For this review, take the finished solid that the model builds, in its own axes (mm). Face numbers are marked on the shaded views. A direction names the side the tool comes from. Round coordinates to 2 decimals unless told otherwise and drop trailing zeros. Write each loop counter-clockwise with the first axis right and the second up, starting at its lowest first coordinate (ties: lowest second). Pieces come first, ordered by that corner, then holes. Notation, with made-up numbers: M 33.5,23 L 39.5,23 A27 ccw 39.5,44 Z; hole C 6.5,59.5 d3. An arc over 180 degrees is marked long. Write each question's results on one line, items separated by ' | '. Start each with the question number.
```python
from build123d import *

# Parameters (mm, degrees)
EXTRUDE1_DEPTH = 7
SHELL1_T       = -1.25
SKETCH2_R      = 2.45
EXTRUDE2_DEPTH = 5.5
EXTRUDE3_REACH = 17.167
SKETCH3_R      = 1.91
EXTRUDE4_REACH = 17.167
SKETCH4_R      = 1.91


with BuildPart() as part:
    # Sketch1 → Extrude1 (new body)
    with BuildSketch(Plane.XY):
        Polygon((-5.45, 6.4), (-7.7, -6.4), (7.7, -6.4), (5.45, 6.4), align=None)
    extrude(amount=EXTRUDE1_DEPTH)

    # Shell1
    shell1_openings = [part.faces().sort_by_distance(p)[0] for p in [
        (0, -6.4, 3.5),
    ]]
    offset(amount=SHELL1_T, openings=shell1_openings, kind=Kind.INTERSECTION)

    # Sketch2 → Extrude2 (add)
    with BuildSketch(Plane(origin=(0, 6.4, 0), x_dir=(1, 0, 0), z_dir=(0, 1, 0))):
        with Locations((0, -3.5)):
            Circle(SKETCH2_R)
    extrude(amount=EXTRUDE2_DEPTH)

    # Sketch3 → Extrude3 (cut, up to next)
    with BuildSketch(Plane(origin=(-6.377928095, 1.121120173, 0), x_dir=(0, 0, 1), z_dir=(-0.984899531, 0.173126871, 0)), mode=Mode.PRIVATE) as extrude3_sk1:
        with Locations((3.5, 1.819815554)):
            Circle(SKETCH3_R)
    extrude3_tool1 = extrude(extrude3_sk1.sketch, amount=-EXTRUDE3_REACH, mode=Mode.PRIVATE) & part.part
    add(extrude3_tool1.solids().sort_by_distance((-6.062869, 2.913456, 3.5))[0], mode=Mode.SUBTRACT)

    # Sketch4 → Extrude4 (cut, up to next)
    with BuildSketch(Plane(origin=(6.377928095, 1.121120173, 0), x_dir=(0, 0, -1), z_dir=(0.984899531, 0.173126871, 0)), mode=Mode.PRIVATE) as extrude4_sk1:
        with Locations((-3.5, 1.819815554)):
            Circle(SKETCH4_R)
    extrude4_tool1 = extrude(extrude4_sk1.sketch, amount=-EXTRUDE4_REACH, mode=Mode.PRIVATE) & part.part
    add(extrude4_tool1.solids().sort_by_distance((6.062869, 2.913456, 3.5))[0], mode=Mode.SUBTRACT)


solid = part.part
```
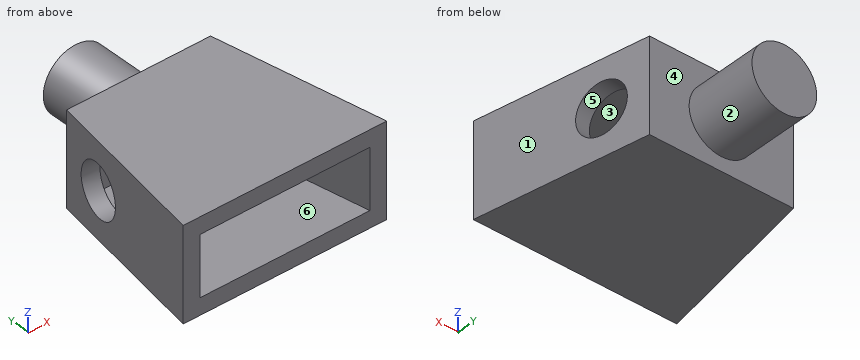
Item 1: Insertion check: P1, Ø4, axis at x = -3, y = 9.5, coming from the -Z side; P2, Ø4, axis at y = 8.5, z = 2, coming from the +X side; P3, Ø2, axis at x = 0, z = 2.5, coming from the -Y side; P4, Ø1, axis at x = 3, y = 8.5, coming from the -Z side. Each pin has a flat end and moves straight along its axis. Give the tip position at first contact, or say it passes through.
Item 2: We need section B-B on y = -1. State the section outline as (x, z) points.
Item 3: We need section C-C on z = 3.5. State the section outline as (x, y) points.
Item 4: We need section A-A on x = 0. State the section outline as (y, z) points.
Item 5: For probe 1 along Z at (x, y) = (-4, 0.5); probe 2 along X at (y, z) = (-2.5, 2.5); probe 3 along X at (y, z) = (0.25, 2), list the stretches that pass through material, from the lowest coordinate up.
Item 6: We need section D-D on x = 4. State the section outline as (y, z) points, then the cut area to 3 significant figures.
Item 7: For the marked faces 4, 5 and 6, list the 3-axis set-ups (+Z, -Z, +X, -X, +Y, -Y) from which the entire face can be reached by the end or side of a thin tool; tool diameter is ignored.
Item 8: Mouldability with a two-part tool opening along X and no side actions: class the marked faces 1, 2 and 3 as pulls with the +X half, pulls with the -X half, needs draft (parallel to the pull), parting line crosses it, or undercut.
Numbers:
1) P1: stops at z = 1.26 | P2: stops at x = 2.45 | P3: stops at y = 5.15 | P4: passes through
2) outline: M -6.75,0 L 6.75,0 L 6.75,7 L -6.75,7 Z; hole M -5.48,1.25 L 5.48,1.25 L 5.48,5.75 L -5.48,5.75 Z
3) outline: M -7.7,-6.4 L -6.43,-6.4 L -5.16,0.82 L -6.39,1.03 Z; M -5.73,4.79 L -4.5,4.58 L -4.4,5.15 L 4.4,5.15 L 4.5,4.58 L 5.73,4.79 L 5.45,6.4 L 2.45,6.4 L 2.45,11.9 L -2.45,11.9 L -2.45,6.4 L -5.45,6.4 Z; M 5.16,0.82 L 6.43,-6.4 L 7.7,-6.4 L 6.39,1.03 Z
4) outline: M -6.4,0 L 6.4,0 L 6.4,1.05 L 11.9,1.05 L 11.9,5.95 L 6.4,5.95 L 6.4,7 L -6.4,7 L -6.4,5.75 L 5.15,5.75 L 5.15,1.25 L -6.4,1.25 Z
5) probe 1: z = 0 to 1.25, 5.75 to 7 | probe 2: x = -7.01 to -5.75, 5.75 to 7.01 | probe 3: x = -6.53 to -5.26, 5.26 to 6.53
6) outline: M -6.4,0 L 6.4,0 L 6.4,7 L -6.4,7 L -6.4,5.75 L 5.15,5.75 L 5.15,1.25 L -6.4,1.25 Z | area: 37.6 mm^2
7) face 4: +Y | face 5: none | face 6: -Y
8) face 1: pulls with the +X half | face 2: parting line crosses it | face 3: undercut
